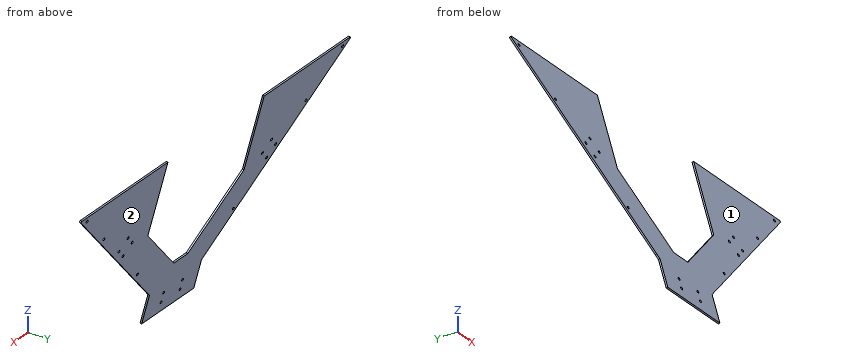
Autodesk Inventor part; units mm, degrees
ref_plane "Work Plane1" through (-1041.8338, 286.0261, 217.3698) normal (0, 0.9659258, -0.258819) x (0.7071068, -0.1830127, -0.6830127)
ref_plane "Work Plane2" through (-962.8473, 265.9096, 142.2942) normal (1, 0, 0) x (0, -0.9659258, 0.258819)
ref_plane "YZ Plane" through (0, 0, 0) normal (1, 0, 0) x (0, 1, 0)
ref_plane "Work Plane1" through (-1041.8338, 286.0261, 217.3698) normal (0, 0.9659258, -0.258819) x (0.7071068, -0.1830127, -0.6830127)
sketch "Sketch1" plane through (-1041.8338, 286.0261, 217.3698) normal (0, 0.9659258, -0.258819) x (0.7071068, -0.1830127, -0.6830127)
  line L0 (110.8111, -517.2111) -> (110.8111, -110.8111) construction
  line L1 (109.9183, -108.6558) -> (2.1553, -0.8927) construction
  line L2 (107.7631, -517.2111) -> (-203.2, -206.248) construction
  line L3 (2.1553, -0.8927) -> (110.8111, -109.5486)
  line L4 (110.8111, -109.5486) -> (110.8111, -517.2111)
  line L5 (110.8111, -517.2111) -> (107.7631, -517.2111)
  line L6 (107.7631, -517.2111) -> (-203.2, -206.248)
  line L7 (56.4832, -55.2206) -> (-148.8721, -260.5759) construction
  line L8 (110.8111, -109.5486) -> (2.1553, -0.8927)
  line L9 (2.1553, -0.8927) -> (-405.5073, -0.8927)
  line L10 (-405.5073, -0.8927) -> (-405.5073, -3.9407)
  line L11 (-405.5073, -3.9407) -> (-94.5442, -314.9038)
  line L12 (110.8111, -109.5486) -> (155.7124, -64.6473)
  line L13 (155.7124, -64.6473) -> (47.0565, 44.0085)
  line L14 (47.0565, 44.0085) -> (2.1553, -0.8927)
  line L15 (2.1553, -0.8927) -> (110.8111, -109.5486)
  point P0 (937.5005, -535.875)
  point P1 (2.1553, -0.8927)
  point P2 (-203.2, -206.248)
  point P3 (110.8111, -109.5486)
  dimension "d1" = 63.5
extrude "Plate1" add sketch "Sketch1" along normal blind 3.048
sketch "Sketch2" plane through (-1041.8338, 288.9702, 216.5809) normal (0, 0.9659258, -0.258819) x (0.7071068, 0.1830127, 0.6830127)
  line L0 (-44.0085, 47.0565) -> (64.6473, 155.7124) construction
  line L1 (64.6473, 155.7124) -> (109.5486, 110.8111) construction
  line L2 (10.3194, 101.3844) -> (24.957, 86.7468) construction
  point P0 (535.875, 937.5005)
  point P1 (42.8728, 104.752)
  point P2 (6.9518, 68.831)
  point P3 (56.3432, 91.2817)
  point P4 (20.4222, 55.3606)
  dimension "d2" = 20.6375
  dimension "d3" = 20.6375
  dimension "d4" = 50.8
  dimension "d7" = 19.05
  dimension "d12" = 25.4
hole "Hole1" at (-937.4473, 277.6455, 174.3166) at (-988.2473, 277.6455, 174.3166) at (-937.4473, 282.576, 192.7175) at (-988.2473, 282.576, 192.7175) direction (0, -0.9659258, 0.258819) diameter 5.1054 end through all
sketch "Sketch3" plane through (-1041.8338, 288.9702, 216.5809) normal (0, 0.9659258, -0.258819) x (0.7071068, 0.1830127, 0.6830127)
  circle A0 centre (56.3432, 91.2817) radius 2.5527 construction
  circle A1 centre (42.8728, 104.752) radius 2.5527 construction
  circle A2 centre (6.9518, 68.831) radius 2.5527 construction
  circle A3 centre (20.4222, 55.3606) radius 2.5527 construction
  line L0 (517.2111, 110.8111) -> (517.2111, 107.7631) construction
  line L1 (109.5486, 110.8111) -> (517.2111, 110.8111) construction
  line L2 (64.6473, 155.7124) -> (109.5486, 110.8111) construction
  line L3 (-44.0085, 47.0565) -> (64.6473, 155.7124) construction
  line L4 (0.8927, 2.1553) -> (-44.0085, 47.0565) construction
  line L5 (0.8927, -405.5073) -> (0.8927, 2.1553) construction
  line L6 (3.9407, -405.5073) -> (0.8927, -405.5073) construction
  line L7 (517.2111, 107.7631) -> (3.9407, -405.5073) construction
  line L8 (10.3194, 101.3844) -> (260.5759, -148.8721) construction
  line L9 (313.3798, 110.8111) -> (313.3798, 98.1111) construction
  line L10 (109.5486, 110.8111) -> (517.2111, 110.8111) construction
  point P0 (535.875, 937.5005)
  point P1 (287.9798, 98.1111)
  point P2 (313.3798, 72.7111)
  point P3 (287.9798, 72.7111)
  point P4 (13.5927, -201.676)
  point P5 (13.5927, -176.276)
  point P6 (38.9927, -201.676)
  point P7 (38.9927, -176.276)
  dimension "d20" = 12.7
  dimension "d23" = 25.4
  dimension "d26" = 25.4
hole "Hole2" at (-750.8658, 328.3671, 363.6122) at (-768.8263, 323.7186, 346.2637) at (-768.8263, 333.0157, 380.9607) at (-786.7868, 328.3671, 363.6122) at (-1156.8682, 333.0157, 380.9607) at (-1138.9077, 328.3671, 363.6122) at (-1174.8287, 328.3671, 363.6122) at (-1156.8682, 323.7186, 346.2637) direction (0, -0.9659258, 0.258819) diameter 5.1054 end through all
sketch "Sketch4" plane through (-1041.8338, 288.9702, 216.5809) normal (0, 0.9659258, -0.258819) x (0.7071068, 0.1830127, 0.6830127)
  line L0 (109.5486, 110.8111) -> (64.6473, 155.7124)
  line L1 (109.5486, 110.8111) -> (100.5683, 110.8111)
  line L2 (109.5486, 110.8111) -> (517.2111, 110.8111)
  line L3 (100.5683, 110.8111) -> (60.1571, 151.2222)
  line L4 (-44.0085, 47.0565) -> (64.6473, 155.7124)
  line L5 (64.6473, 155.7124) -> (60.1571, 151.2222)
  point P0 (535.875, 937.5005)
  dimension "d36" = 6.35
extrude "Cut1" cut sketch "Sketch4" against normal blind 3.048
ref_plane "Work Plane2" through (-962.8473, 265.9096, 142.2942) normal (1, 0, 0) x (0, -0.9659258, 0.258819)
mirror "Mirror1" about plane through (-962.8473, 265.9096, 142.2942) normal (1, 0, 0) of "Cut1"
sketch "Sketch5" plane through (-1041.8338, 288.9702, 216.5809) normal (0, 0.9659258, -0.258819) x (0.7071068, 0.1830127, 0.6830127)
  line L0 (100.5683, 110.8111) -> (517.2111, 110.8111)
  line L1 (517.2111, 101.9084) -> (109.471, 101.9084) construction
  line L2 (517.2111, 110.8111) -> (517.2111, 107.7631)
  line L3 (100.5683, 110.8111) -> (60.1571, 151.2222)
  point P0 (535.875, 937.5005)
  point P1 (498.1611, 101.9084)
  point P2 (396.5611, 101.9084)
  point P3 (193.3611, 101.9084)
  dimension "d40" = 8.9027
  dimension "d41" = 101.6
  dimension "d42" = 19.05
  dimension "d45" = 203.2
hole "Hole3" at (-617.5206, 361.4895, 487.2266) at (-689.3626, 342.8954, 417.8325) at (-833.0467, 305.7072, 279.0443) direction (0, -0.9659258, 0.258819) diameter 5.1054 end through all
mirror "Mirror2" about plane through (-962.8473, 265.9096, 142.2942) normal (1, 0, 0) of "Hole3"
sketch "Sketch8" plane through (-1041.8338, 288.9702, 216.5809) normal (0, 0.9659258, -0.258819) x (0.7071068, 0.1830127, 0.6830127)
  line L0 (352.6003, -56.8477) -> (248.4416, 47.3111)
  line L1 (248.4416, 47.3111) -> (91.3335, 47.3111)
  line L2 (64.3927, 20.3703) -> (64.3927, -136.7378)
  line L3 (64.3927, -136.7378) -> (168.5515, -240.8965)
  line L4 (0.8927, 11.1355) -> (0.8927, -405.5073)
  line L5 (100.5683, 110.8111) -> (517.2111, 110.8111)
  line L6 (517.2111, 107.7631) -> (3.9407, -405.5073)
  line L7 (-39.5184, 51.5467) -> (60.1571, 151.2222) construction
  line L8 (10.3194, 101.3844) -> (260.5759, -148.8721) construction
  line L9 (64.3927, 20.3703) -> (91.3335, 47.3111)
  point P0 (535.875, 937.5005)
  point P1 (64.3927, -58.1837)
  dimension "d62" = 63.5
  dimension "d65" = 234.95
  dimension "d66" = 234.95
  dimension "d75" = 63.5
  dimension "d76" = 135
  dimension "d77" = 135
extrude "Extrusion2" cut sketch "Sketch8" against normal blind 25.4
equation "\"d18\" = Thickness"
equation "\"d37\" = Thickness"
equation "\"d51\" = Thickness"
equation "\"d0\" = Thickness"
equation "\"BendRadius\" = Thickness"
equation "\"BendReliefWidth\" = Thickness"
equation "\"BendReliefDepth\" = 0.5 * Thickness"
equation "\"CornerReliefSize\" = 4 * Thickness"
equation "\"MinimumRemnant\" = 2 * Thickness"
equation "\"TransitionRadius\" = BendRadius"
equation "\"JacobiRadiusSize\" = BendRadius"
equation "\"GapSize\" = Thickness"
properties part number "hopper_back" material "Polycarbonate, Clear"
Verification items for the finished model (mm, model axes). Face numbers are marked on the shaded views. Round coordinates to 2 decimals unless told otherwise and drop trailing zeros. Loops run counter-clockwise (first coordinate to the right, second up) from the corner with the lowest first, then second, coordinate; pieces in that order, holes last. Notation, with made-up numbers: (15, -2) - (29, -2) arc R24 cw to (29, 16) - close; hole circle Ø8 at (47.25, 9.5). An arc over 180 degrees is marked (long way). Answer in a Markdown table with one row per item. Add a question column.
Q1. Section check D-D on x = -1256.5. Enter the section's corners in (y, z).
Q2. Section check A-A on z = 473. Enter the section's corners in (x, y), plus the area to 3 significant figures.
Q3. Gauge pin test, flat ends, axial feed: pin 1 (12 mm diameter, centred on x = -840, z = 261, fed in from +Y); pin 2 (19.5 mm diameter, centred on y = 274, z = 189, fed in from -X); pin 3 (14 mm diameter, centred on y = 282, z = 179, fed in from +X). Record the tip position at first contact, or that the pin passes through.
Q4. Release check for a two-part mould opening along Z. For the marked faces 1 and 2 record: pulls with the +Z half, pulls with the -Z half, needs draft (parallel to the pull), parting line crosses it, or undercut.
Q5. Section check C-C on z = 319. Enter the section's corners in (x, y), plus the area to 3 significant figures.
Q6. Section check B-B on x = -923.5. Enter the section's corners in (y, z), plus the area to 3 significant figures.
Q7. Material ranges on line 1 (Y direction, x = -1287, z = 479.5); line 2 (Y direction, x = -787, z = 463), recorded low to high.
Found:
| question | item | result |
|---|---|---|
| 1 | outline | (341.91, 425.94) - (344.86, 425.15) - (363.9, 496.24) - (360.96, 497.03) - close |
| 2 | outline | (-1306.04, 357.68) - (-1305.22, 354.52) - (-1092.99, 354.52) - (-1092.99, 357.68) - close; (-832.71, 354.52) - (-620.48, 354.52) - (-619.66, 357.68) - (-832.71, 357.68) - close |
| 2 | area | 1,340 mm² |
| 3 | pin 1 | stops at y = 302.48 |
| 3 | pin 2 | stops at x = -1033.33 |
| 3 | pin 3 | stops at x = -892.37 |
| 4 | face 1 | pulls with the +Z half |
| 4 | face 2 | pulls with the -Z half |
| 5 | outline | (-1146.6, 316.41) - (-1145.79, 313.26) - (-1055.98, 313.26) - (-1056.8, 316.41) - close; (-869.71, 313.26) - (-779.91, 313.26) - (-779.09, 316.41) - (-868.89, 316.41) - close |
| 5 | area | 567 mm² |
| 6 | outline | (269.36, 155.17) - (272.3, 154.38) - (302.28, 266.25) - (299.34, 267.04) - close |
| 6 | area | 353 mm² |
| 7 | line 1 | y = 356.26 to 359.42 |
| 7 | line 2 | y = 351.84 to 355 |
